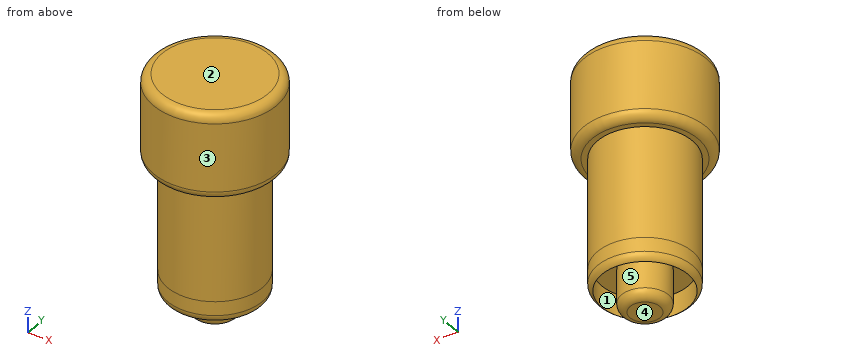
Autodesk Inventor part; units mm, degrees
ref_plane "YZ Plane" through (0, 0, 0) normal (1, 0, 0) x (0, 1, 0)
ref_plane "XZ Plane" through (0, 0, 0) normal (0, 1, 0) x (-1, 0, 0)
ref_plane "XY Plane" through (0, 0, 0) normal (0, 0, 1) x (1, 0, 0)
sketch "Sketch1" plane through (0, 0, 0) normal (0, 0, 1) x (1, 0, 0)
  circle A0 centre (0, 0) radius 5.5
  dimension "d0" = 11
extrude "Extrusion1" add sketch "Sketch1" along normal blind 10
sketch "Sketch2" plane through (0, 0, 10) normal (0, 0, 1) x (1, 0, 0)
  circle A0 centre (0, 0) radius 11.15
  dimension "d3" = 22.3
extrude "Extrusion3" add sketch "Sketch2" along normal blind 26
sketch "Sketch3" plane through (0, 0, 10) normal (0, 0, -1) x (-1, 0, 0)
  circle A0 centre (0, 0) radius 10.15
  circle A1 centre (0, 0) radius 11.15
  dimension "d8" = 20.3
  dimension "d9" = 22.3
extrude "Extrusion4" add sketch "Sketch3" along normal blind 5
sketch "Sketch4" plane through (0, 0, 36) normal (0, 0, 1) x (1, 0, 0)
  circle A0 centre (0, 0) radius 14.45
  dimension "d12" = 28.9
extrude "Extrusion5" add sketch "Sketch4" along normal blind 20
fillet "Fillet1" radius 2 1 edges at (-14.45, 0, 56)
fillet "Fillet2" radius 2 1 edges at (-5.5, 0, 0)
fillet "Fillet3" radius 2 1 edges at (11.15, 0, 5)
fillet "Fillet4" radius 2 1 edges at (-14.45, 0, 36)
properties part number "Elbow_Parallel_Rod_V1"
Work out the finished part from the listing and answer in its coordinate system (mm). Face numbers are marked on the shaded views. A direction names the side the tool comes from. Give positions to 0.01 mm unless a question says otherwise; leave off trailing zeros. Loops run counter-clockwise (first coordinate to the right, second up) from the corner with the lowest first, then second, coordinate; pieces in that order, holes last. Notation, with made-up numbers: (75.5, 63) - (98.5, 63) arc R22 cw to (98.5, 93) - close; hole circle Ø6 at (81.5, 54). An arc over 180 degrees is marked (long way). Use CSV: the item, a comma, the result in double quotes. Start each with the question number.
(1) A tool of negligible diameter and unlimited length cuts with its end or side. For the marked faces 4 and 5, from which of +Z, -Z, +X, -X, +Y, -Y can it reach the whole face along a straight path? Write none if from no direction.
(2) Find section D-D, the plane z = 34.5. Determine the outline of the cut face in (x, y), plus the area to 3 significant figures.
(3) Each of these flat-tipped pins is pushed along its axis until it touches: pin 1 (5 mm diameter, centred on y = 8, z = 20, fed in from -X); pin 2 (6 mm diameter, centred on y = -11, z = 34.5, fed in from +X); pin 3 (12 mm diameter, centred on y = 11, z = 6.5, fed in from +X). Where does it stop, or does it pass through?
(4) Find section C-C, the plane z = 42. Determine the outline of the cut face in (x, y).
(5) Find the intervals of material crossed by L1, parallel to Y at x = 0, z = 6.25; L2, parallel to X at y = 0.75, z = 8; L3, parallel to Y at x = 0, z = 6.1, in increasing order.
(6) Determine the mould class of the marked faces 1, 2 and 3 for opening direction X: released by +X, released by -X, zero draft, split by the parting line, or undercut.
(7) Find section A-A, the plane y = 0. Determine the outline of the cut face in (x, z), plus the area to 3 significant figures.
Results found:
1,face 4,"-Z, +X, -X, +Y, -Y"
1,face 5,"-Z"
2,outline,"circle Ø22.3 at (0, 0)"
2,area,"391 mm^2"
3,pin 1,"x = -9.7"
3,pin 2,"x = 10.73"
3,pin 3,"x = 9.96"
4,outline,"circle Ø28.9 at (0, 0)"
5,L1,"-11.09 to -10.15, -5.5 to 5.5, 10.15 to 11.09"
5,L2,"-11.12 to -10.12, -5.45 to 5.45, 10.12 to 11.12"
5,L3,"-11.05 to -10.15, -5.5 to 5.5, 10.15 to 11.05"
6,face 1,"undercut"
6,face 2,"zero draft"
6,face 3,"split by the parting line"
7,outline,"(-14.45, 38) arc R2 ccw to (-12.45, 36) - (-11.15, 36) - (-11.15, 6.73) arc R2 ccw to (-10.15, 5) - (-10.15, 10) - (-5.5, 10) - (-5.5, 2) arc R2 ccw to (-3.5, 0) - (3.5, 0) arc R2 ccw to (5.5, 2) - (5.5, 10) - (10.15, 10) - (10.15, 5) arc R2 ccw to (11.15, 6.73) - (11.15, 36) - (12.45, 36) arc R2 ccw to (14.45, 38) - (14.45, 54) arc R2 ccw to (12.45, 56) - (-12.45, 56) arc R2 ccw to (-14.45, 54) - close"
7,area,"1,270 mm^2"
